from build123d import *

# Parameters (mm, degrees)
SKETCH1_R                               = 8.477787946
BOSS_EXTRUDE1_DEPTH                     = 6
SKETCH2_R                               = 1.75
CUT_EXTRUDE1_DEPTH                      = 3
CBORE_FOR_M5_HEX_HEAD_BOLT1_D           = 1.5
CBORE_FOR_M5_HEX_HEAD_BOLT1_CBORE_D     = 4
CBORE_FOR_M5_HEX_HEAD_BOLT1_CBORE_DEPTH = 1
CUT_EXTRUDE6_START                      = -1.48
SKETCH10_W                              = 21.455120181
SKETCH10_H                              = 4
CUT_EXTRUDE6_DEPTH                      = 4
SKETCH12_W                              = 22.336955322
SKETCH12_H                              = 4
CUT_EXTRUDE7_DEPTH                      = 4
SKETCH13_R                              = 1
CUT_EXTRUDE8_DEPTH                      = 4


with BuildPart() as part:
    # Sketch1 → Boss-Extrude1 (new body)
    with BuildSketch(Plane(origin=(0, 0, 0), x_dir=(1, 0, 0), z_dir=(0, 1, 0))):
        with Locations(Location((-4.607856835, 9.967667798, 0), (0, 0, 270))):
            Circle(SKETCH1_R)
    extrude(amount=-BOSS_EXTRUDE1_DEPTH)

    # Sketch2 → Cut-Extrude1 (cut)
    with BuildSketch(Plane(origin=(0, 0, 0), x_dir=(1, 0, 0), z_dir=(0, 1, 0))):
        with Locations(Location((-10.434250808, 9.967667798, 0), (0, 0, 270))):
            Circle(SKETCH2_R)
        with Locations(Location((1.218537138, 9.967667798, 0), (0, 0, 270))):
            Circle(SKETCH2_R)
    extrude(amount=-CUT_EXTRUDE1_DEPTH, mode=Mode.SUBTRACT)

    # CBORE for M5 Hex Head Bolt1 (through all)
    with Locations(Plane(origin=(0, -6, 0), x_dir=(-1, 0, 0), z_dir=(0, -1, 0))):
        with Locations((10.434250808, 9.967667798), (-1.218537138, 9.967667798)):
            CounterBoreHole(CBORE_FOR_M5_HEX_HEAD_BOLT1_D / 2, CBORE_FOR_M5_HEX_HEAD_BOLT1_CBORE_D / 2, CBORE_FOR_M5_HEX_HEAD_BOLT1_CBORE_DEPTH)

    # Sketch10 → Cut-Extrude6 (cut)
    with BuildSketch(Plane.XY.offset(CUT_EXTRUDE6_START)):
        with Locations((-4.34718715, -3)):
            Rectangle(SKETCH10_W, SKETCH10_H)
    extrude(amount=-CUT_EXTRUDE6_DEPTH, mode=Mode.SUBTRACT)

    # Sketch12 → Cut-Extrude7 (cut)
    with BuildSketch(Plane(origin=(0, 0, -18.445455745), x_dir=(-1, 0, 0), z_dir=(0, 0, -1))):
        with Locations((4.129052905, -3)):
            Rectangle(SKETCH12_W, SKETCH12_H)
    extrude(amount=-CUT_EXTRUDE7_DEPTH, mode=Mode.SUBTRACT)

    # Sketch13 → Cut-Extrude8 (cut)
    with BuildSketch(Plane(origin=(0, 0, 0), x_dir=(1, 0, 0), z_dir=(0, 1, 0))):
        with Locations((1.886505511, 4.518250749)):
            Circle(SKETCH13_R)
        with Locations((-11.102219182, 4.518250749)):
            Circle(SKETCH13_R)
        with Locations((-11.102219182, 15.417084848)):
            Circle(SKETCH13_R)
        with Locations((1.886505511, 15.417084848)):
            Circle(SKETCH13_R)
    extrude(amount=-CUT_EXTRUDE8_DEPTH, mode=Mode.SUBTRACT)


solid = part.part
Design review of the part built by this model. Coordinates are the model's own, in mm. A direction names the side the tool comes from. Coordinates: 2 decimals unless noted, no trailing zeros. Loops run counter-clockwise (first coordinate to the right, second up) from the corner with the lowest first, then second, coordinate; pieces in that order, holes last.
Item 1: Clearance check with flat-ended pins moving along their axes: pin 1 (2 mm diameter, centred on x = -10.43, z = -9.97, fed in from +Y); pin 2 (2.5 mm diameter, centred on x = 1.22, z = -9.97, fed in from -Y); pin 3 (1 mm diameter, centred on y = -4, z = -8.5, fed in from +X). State where each tip first meets the part, or that it passes through.
Completed:
pin 1: stops at y = -3
pin 2: stops at y = -5
pin 3: stops at x = 3.81
Item 2: Add section C-C (x = -3.75). Write out the cut boundary in (y, z), and give its area (3 significant figures).
Completed:
outline: (-6, -18.4) - (-5, -18.4) - (-5, -14.45) - (-1, -14.45) - (-1, -18.4) - (0, -18.4) - (0, -1.53) - (-1, -1.53) - (-1, -5.48) - (-5, -5.48) - (-5, -1.53) - (-6, -1.53) - close
area: 69.6 mm2
Item 3: Add section D-D (z = -7.75). Write out the cut boundary in (x, y), and give its area (3 significant figures).
Completed:
outline: (-12.79, -6) - (3.57, -6) - (3.57, 0) - (-12.79, 0) - close
area: 98.2 mm2
Item 4: Wall thickness on L1, parallel to Y at x = -5.5, z = -17.5; L2, parallel to X at y = -1.2, z = -9.5; L3, parallel to Y at x = -11.25, z = -14.75: over which ranges is each line inside the solid? List them lowest first.
Completed:
L1: y = -6 to -5, -1 to 0
L2: x = -13.07 to -12.12, -8.75 to -0.47, 2.9 to 3.86
L3: y = -6 to -5
Item 5: Add section A-A (z = -9.75). Write out the cut boundary in (x, y).
Completed:
outline: (-13.08, -6) - (-12.42, -6) - (-12.42, -5) - (-11.15, -5) - (-11.15, -3) - (-12.17, -3) - (-12.17, 0) - (-13.08, 0) - close; (-9.72, -5) - (-8.45, -5) - (-8.45, -6) - (-0.77, -6) - (-0.77, -5) - (0.5, -5) - (0.5, -3) - (-0.52, -3) - (-0.52, 0) - (-8.7, 0) - (-8.7, -3) - (-9.72, -3) - close; (1.94, -5) - (3.21, -5) - (3.21, -6) - (3.87, -6) - (3.87, 0) - (2.95, 0) - (2.95, -3) - (1.94, -3) - close
Item 6: Add section B-B (y = -3.4). Write out the cut boundary in (x, z), and give its area (3 significant figures).
Completed:
outline: (-11.81, -14.45) - (-11.34, -14.45) arc R1 cw to (-10.87, -14.45) - (1.65, -14.45) arc R1 cw to (2.12, -14.45) - (2.59, -14.45) arc R8.48 ccw to (2.58, -5.48) - (2.16, -5.48) arc R1 cw to (1.61, -5.48) - (-10.83, -5.48) arc R1 cw to (-11.38, -5.48) - (-11.8, -5.48) arc R8.48 ccw to start; hole circle Ø1.5 at (-10.43, -9.97); hole circle Ø1.5 at (1.22, -9.97)
area: 141 mm2
Item 7: Draft analysis for pull direction Z (two halves, no side actions). For faces 1 (the cylindrical face through (1.652, -5.507, -8.015)), 2 (the cylindrical face through (-12.13, -2.96, -6.06)), 3 (the flat face through (-4, 0, -10)), state which applies: pulls with the +Z half, pulls with the -Z half, needs draft (parallel to the pull), parting line crosses it, or undercut.
Completed:
face 1: undercut
face 2: parting line crosses it
face 3: needs draft
Item 8: For faces 4 (the flat face through (-5, -5, -4)), 5 (the cylindrical face through (-8.85, -5.51, -8.75)), 6 (the cylindrical face through (1.744, -1.479, -8.298)), list the 3-axis set-ups (+Z, -Z, +X, -X, +Y, -Y) from which the entire face can be reached by the end or side of a thin tool; tool diameter is ignored.
Completed:
face 4: +Z, +X, -X
face 5: -Y
face 6: +Y
